from build123d import *

# Parameters (mm, degrees)
SKETCH1_W           = 6.35
SKETCH1_H           = 40
SKETCH1_W_2         = 360
SKETCH1_H_2         = 300
BOSS_EXTRUDE1_DEPTH = 6.35


with BuildPart() as part:
    # Sketch1 → Boss-Extrude1 (new body)
    with BuildSketch(Plane.XY):
        Polygon((0, 0), (420, 0), (420, 457.5), (413.65, 457.5), (407.3, 457.5), (12.7, 457.5), (6.35, 457.5), (0, 457.5), align=None)
        with Locations((9.525, 385)):
            Rectangle(SKETCH1_W, SKETCH1_H, mode=Mode.SUBTRACT)
        with Locations((410.475, 385)):
            Rectangle(SKETCH1_W, SKETCH1_H, mode=Mode.SUBTRACT)
        with Locations((9.525, 230)):
            Rectangle(SKETCH1_W, SKETCH1_H, mode=Mode.SUBTRACT)
        with Locations((410.475, 230)):
            Rectangle(SKETCH1_W, SKETCH1_H, mode=Mode.SUBTRACT)
        with Locations((410.475, 75)):
            Rectangle(SKETCH1_W, SKETCH1_H, mode=Mode.SUBTRACT)
        with Locations((9.525, 75)):
            Rectangle(SKETCH1_W, SKETCH1_H, mode=Mode.SUBTRACT)
        with Locations((210, 195)):
            Rectangle(SKETCH1_W_2, SKETCH1_H_2, mode=Mode.SUBTRACT)
    extrude(amount=BOSS_EXTRUDE1_DEPTH)


solid = part.part
Verification items for the finished model (mm, model axes). Coordinates: 2 decimals unless noted, no trailing zeros. Order: outer loops, then holes, each group sorted by start corner. A loop starts at its lowest first (then second) coordinate and runs counter-clockwise, first axis right, second up. Notation, with made-up numbers: M -35.75,46 L 15.25,46 A24 cw 15.25,81 Z; hole C -38,85 d3. An arc over 180 degrees is marked long. Return JSON: item names as keys, results as strings.
1) Cross-section at A-A, the plane x = 350. Record the boundary of the cut face in (y, z).
Answer list:
{"outline": "M 0,0 L 45,0 L 45,6.35 L 0,6.35 Z; M 345,0 L 457.5,0 L 457.5,6.35 L 345,6.35 Z"}
2) Cross-section at B-B, the plane y = 315. Record the boundary of the cut face in (x, z), and give its area (3 significant figures).
Answer list:
{"outline": "M 0,0 L 30,0 L 30,6.35 L 0,6.35 Z; M 390,0 L 420,0 L 420,6.35 L 390,6.35 Z", "area": "381 mm2"}
3) Thickness scan on L1, parallel to X at y = 399.5, z = 1; L2, parallel to X at y = 73, z = 3; L3, parallel to X at y = 301, z = 1. Record the ranges inside material, lowest first. Write a range as [from, to].
Answer list:
{"L1": "[0, 6.35], [12.7, 407.3], [413.65, 420]", "L2": "[0, 6.35], [12.7, 30], [390, 407.3], [413.65, 420]", "L3": "[0, 30], [390, 420]"}
4) Cross-section at C-C, the plane z = 5. Count the separate pieces of the cut face and the enclosed holes in it, and give its area (3 significant figures).
Answer list:
{"separate pieces": "1", "enclosed holes": "7", "area": "82,600 mm2"}
5) Gauge pin test, flat end, axial feed: pin 1 (3 mm diameter, centred on x = 9.5, z = 2.5, fed in from -Y). Record the tip position at first contact, or that the pin passes through.
Answer list:
{"pin 1": "y = 0"}
